For this review, take the finished solid that the model builds, in its own axes (mm). Give positions to 0.01 mm unless a question says otherwise; leave off trailing zeros. Order: outer loops, then holes, each group sorted by start corner. A loop starts at its lowest first (then second) coordinate and runs counter-clockwise, first axis right, second up.
Item 1: For probe 1 along X at (y, z) = (-4.5, 0.55); probe 2 along Y at (x, z) = (25.21, 0.25); probe 3 along Y at (x, z) = (31.21, 0.55), list the stretches that pass through material, from the lowest coordinate up.
Item 2: Consider section C-C (y = -41.5). Give the boundary of the cut face in (x, z) (3 decimals).
Item 3: Consider section A-A (x = 25.21). Give the boundary of the cut face in (y, z).
Item 4: Consider section D-D (z = 0.6). Give the number of separate pieces and of enclosed holes in the cut face, plus the area to 3 significant figures.
Item 5: Consider section B-B (x = 31.21). Give the boundary of the cut face in (y, z), plus the area to 3 significant figures.
Item 6: For P1, Ø5, axis at x = 11.5, y = -4.5, coming from the -Z side; P2, Ø0.5, axis at y = 0.5, z = 0.5, coming from the -X side; P3, Ø0.5, axis at x = 3, z = 0.5, coming from the -Y side; P4, Ø0.5, axis at y = 0.5, z = 0.5, coming from the +X side, all flat-tipped, find the tip position at first contact; note any pin that passes through.
```python
from build123d import *

# Parameters (mm, degrees)
BOSS_EXTRUDE2_DEPTH = 1
SKETCH2_R           = 1.5
SKETCH2_R_2         = 1.499999993
CUT_EXTRUDE8_DEPTH  = 3
FILLET2_R           = 4
FILLET3_R           = 5
FILLET4_R           = 4
FILLET5_R           = 5
FILLET6_R           = 2
FILLET7_R           = 2
FILLET8_R           = 2
FILLET9_R           = 2
FILLET12_R          = 4
FILLET13_R          = 5


with BuildPart() as part:
    # Sketch1 → Boss-Extrude2 (new body)
    with BuildSketch(Plane.XY):
        Polygon((0, 0), (4.18, 0), (4.18, 1), (12.43, 1), (12.43, 0), (24.28, 0), (24.28, 1), (32.53, 1), (32.53, 0), (36.71, 0), (36.71, -11.5), (27.585, -11.5), (27.585, -86.5), (36.71, -86.5), (36.71, -98), (32.53, -98), (32.53, -99), (24.28, -99), (24.28, -98), (12.43, -98), (12.43, -99), (4.18, -99), (4.18, -98), (0, -98), (0, -86.5), (9.125, -86.5), (9.125, -11.5), (0, -11.5), align=None)
    extrude(amount=BOSS_EXTRUDE2_DEPTH)

    # Sketch2 → Cut-Extrude8 (cut)
    with BuildSketch(Plane.XY):
        with Locations((5.5, -4.499987612)):
            Circle(SKETCH2_R)
        with Locations((11.5, -4.499987612)):
            Circle(SKETCH2_R)
        with Locations((25.21, -4.5)):
            Circle(SKETCH2_R)
        with Locations((31.21, -4.5)):
            Circle(SKETCH2_R_2)
        with Locations((5.5, -93.500004994)):
            Circle(SKETCH2_R)
        with Locations((11.5, -93.500004994)):
            Circle(SKETCH2_R)
        with Locations((25.21, -93.5)):
            Circle(SKETCH2_R)
        with Locations((31.21, -93.5)):
            Circle(SKETCH2_R)
    extrude(amount=CUT_EXTRUDE8_DEPTH, mode=Mode.SUBTRACT)

    # Fillet2
    fillet2_edges = [part.edges().sort_by_distance(p)[0] for p in [
        (36.71, -86.5, 0.5),
    ]]
    fillet(fillet2_edges, radius=FILLET2_R)

    # Fillet3
    fillet3_edges = [part.edges().sort_by_distance(p)[0] for p in [
        (27.585, -86.5, 0.5),
    ]]
    fillet(fillet3_edges, radius=FILLET3_R)

    # Fillet4
    fillet4_edges = [part.edges().sort_by_distance(p)[0] for p in [
        (0, -86.5, 0.5),
    ]]
    fillet(fillet4_edges, radius=FILLET4_R)

    # Fillet5
    fillet5_edges = [part.edges().sort_by_distance(p)[0] for p in [
        (9.125, -86.5, 0.5),
    ]]
    fillet(fillet5_edges, radius=FILLET5_R)

    # Fillet6
    fillet6_edges = [part.edges().sort_by_distance(p)[0] for p in [
        (0, -98, 0.5),
    ]]
    fillet(fillet6_edges, radius=FILLET6_R)

    # Fillet7
    fillet7_edges = [part.edges().sort_by_distance(p)[0] for p in [
        (36.71, -98, 0.5),
    ]]
    fillet(fillet7_edges, radius=FILLET7_R)

    # Fillet8
    fillet8_edges = [part.edges().sort_by_distance(p)[0] for p in [
        (0, 0, 0.5),
    ]]
    fillet(fillet8_edges, radius=FILLET8_R)

    # Fillet9
    fillet9_edges = [part.edges().sort_by_distance(p)[0] for p in [
        (36.71, 0, 0.5),
    ]]
    fillet(fillet9_edges, radius=FILLET9_R)

    # Fillet12
    fillet12_edges = [part.edges().sort_by_distance(p)[0] for p in [
        (36.71, -11.5, 0.5),
        (0, -11.5, 0.5),
    ]]
    fillet(fillet12_edges, radius=FILLET12_R)

    # Fillet13
    fillet13_edges = [part.edges().sort_by_distance(p)[0] for p in [
        (27.585, -11.5, 0.5),
        (9.125, -11.5, 0.5),
    ]]
    fillet(fillet13_edges, radius=FILLET13_R)


solid = part.part
```
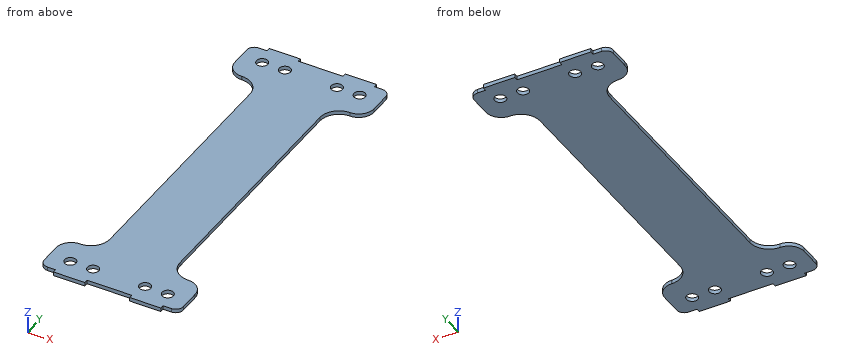
Resolved:
1. probe 1: x = 0 to 4, 7 to 10, 13 to 23.71, 26.71 to 29.71, 32.71 to 36.71
1. probe 2: y = -99 to -95, -92 to -6, -3 to 1
1. probe 3: y = -99 to -95, -92 to -86.31, -11.69 to -6, -3 to 1
2. outline: (9.125, 0) - (27.585, 0) - (27.585, 1) - (9.125, 1) - close
3. outline: (-99, 0) - (-95, 0) - (-95, 1) - (-99, 1) - close; (-92, 0) - (-6, 0) - (-6, 1) - (-92, 1) - close; (-3, 0) - (1, 0) - (1, 1) - (-3, 1) - close
4. separate pieces: 1
4. enclosed holes: 8
4. area: 2,210 mm2
5. outline: (-99, 0) - (-95, 0) - (-95, 1) - (-99, 1) - close; (-92, 0) - (-86.31, 0) - (-86.31, 1) - (-92, 1) - close; (-11.69, 0) - (-6, 0) - (-6, 1) - (-11.69, 1) - close; (-3, 0) - (1, 0) - (1, 1) - (-3, 1) - close
5. area: 19.4 mm2
6. P1: stops at z = 0
6. P2: stops at x = 4.18
6. P3: stops at y = -98
6. P4: stops at x = 32.53
